from build123d import *

# Parameters (mm, degrees)
BOSS_EXTRUDE1_DEPTH     = 12.7
FILLET2_SIZE            = 41.275
FILLET2_SIZE_2          = 69.85
FILLET3_R               = 25.4
FILLET4_R               = 19.05
FILLET5_START           = -1
FILLET5_DEPTH           = 15
FILLET6_R               = 127
CUT_EXTRUDE1_REACH      = 634.314
SKETCH3_W               = 241.600142069
SKETCH3_H               = 584.2
F_8_CLEARANCE_HOLE1_D   = 4.9149
F_1_4_CLEARANCE_HOLE1_D = 7.14248


with BuildPart() as part:
    # Sketch1 → Boss-Extrude1 (new body)
    with BuildSketch(Plane.XY):
        Polygon((-228.088766336, 0), (228.088766336, 0), (228.088766336, -443.878997916), (241.600142069, -584.2), (237.284597128, -584.2), (202.688766336, -463.55), (79.375, -463.55), (79.375, -363.22), (-79.375, -363.22), (-79.375, -463.55), (-202.688766336, -463.55), (-237.284597128, -584.2), (-241.600142069, -584.2), (-228.088766336, -443.878997916), align=None)
    extrude(amount=BOSS_EXTRUDE1_DEPTH)

    # Fillet2
    # a fillet whose section is not a circle: 69.85, 41.275 mm, written as the material it adds along each edge
    with BuildSketch(Plane(origin=(-79.375, -363.22, 0), x_dir=(1, 0, 0), z_dir=(0, 0, 1))) as fillet2_piece_1:
        with BuildLine():
            Bezier((FILLET2_SIZE, 0), (0, 0), (0, -FILLET2_SIZE_2), weights=[1, 1.5, 1])
            Line((0, -FILLET2_SIZE_2), (0, 0))
            Line((0, 0), (FILLET2_SIZE, 0))
        make_face()
    extrude(amount=12.7)

    # Fillet3
    fillet3_edges = [part.edges().sort_by_distance(p)[0] for p in [
        (-79.375, -463.55, 6.35),
    ]]
    fillet(fillet3_edges, radius=FILLET3_R)

    # Fillet4
    fillet4_edges = [part.edges().sort_by_distance(p)[0] for p in [
        (-202.688766336, -463.55, 6.35),
    ]]
    fillet(fillet4_edges, radius=FILLET4_R)

    # Fillet5: read off the stored shape, not the designer's step
    # Fillet5 outline → Fillet5 (cut)
    with BuildSketch(Plane.XY.offset(FILLET5_START)):
        with BuildLine():
            Line((-237.284597128, -584.2), (-224.526592015, -539.707548693))
            add(Edge.make_bspline(
                [(-224.526592015, -539.707548693), (-237.177095318, -583.825096633), (-241.600142069, -584.2)],
                knots=[0, 0, 0, 1, 1, 1], degree=2, weights=[1, 2.333333333, 1]))
            Line((-241.600142069, -584.2), (-237.284597128, -584.2))
        make_face()
    extrude(amount=FILLET5_DEPTH, mode=Mode.SUBTRACT)

    # Fillet6
    # the kernel refuses this fillet: 127 mm, written as the material it adds along each edge
    with BuildSketch(Plane(origin=(-228.088766336, -443.878997916, 0), x_dir=(0, 1, 0), z_dir=(0, 0, 1))) as fillet6_piece_1:
        with BuildLine():
            CenterArc((FILLET6_R * 0.0480334444852, FILLET6_R), FILLET6_R, 264.5, 5.5)
            Line((-FILLET6_R * 0.047812308035, FILLET6_R * 0.00460380163282), (0, 0))
            Line((0, 0), (FILLET6_R * 0.0480334444852, 0))
        make_face()
    extrude(amount=12.7)

    # Sketch3 → Cut-Extrude1 (cut, up to next)
    with BuildSketch(Plane.XY.offset(12.7), mode=Mode.PRIVATE) as cut_extrude1_sk1:
        with Locations((120.800071035, -292.1)):
            Rectangle(SKETCH3_W, SKETCH3_H)
    cut_extrude1_tool1 = extrude(cut_extrude1_sk1.sketch, amount=-CUT_EXTRUDE1_REACH, mode=Mode.PRIVATE) & part.part
    add(cut_extrude1_tool1.solids().sort_by_distance((120.800071, -292.1, 12.7))[0], mode=Mode.SUBTRACT)

    # Mirror5: part across plane


with BuildPart() as part_1:
    add(part.part)
    add(part.part.mirror(Plane(origin=(0, 0, -0.35025), x_dir=(0, 0, 1), z_dir=(-1, 0, 0))))

    # #8 Clearance Hole1 (through all)
    with Locations(Plane(origin=(0, 0, 0), x_dir=(-1, 0, 0), z_dir=(0, 0, -1))):
        with Locations((12.077216058, -342.5825), (-12.077216058, -342.5825)):
            Hole(F_8_CLEARANCE_HOLE1_D / 2)

    # 1/4 Clearance Hole1 (through all)
    with Locations(Plane(origin=(0, 0, 0), x_dir=(-1, 0, 0), z_dir=(0, 0, -1))):
        with Locations((0, -352.7425), (0, -332.4225)):
            Hole(F_1_4_CLEARANCE_HOLE1_D / 2)


solid = part_1.part
Input: part model. Units: mm. Frame: model coordinates. A direction names the side the tool comes from. Coordinates: 2 decimals unless noted, no trailing zeros. Order: outer loops, then holes, each group sorted by start corner. A loop starts at its lowest first (then second) coordinate and runs counter-clockwise, first axis right, second up. Notation, with made-up numbers: M 30,56.25 L 43,56.25 A24 cw 43,85.25 Z; hole C 72,-39 d7. An arc over 180 degrees is marked long. Answer as CSV lines item,"result".
1. Access query for faces 4 (the cylindrical face through (199.66, -467.283, 6.439)), 5 (the flat face through (228.089, -222, 6)), 6 (the flat face through (3, -223, 0)). Directions: +Z, -Z, +X, -X, +Y, -Y. A direction counts if a zero-diameter tool reaches every point of the face in a straight line with its end or side. Return the directions, or none.
Reported:
face 4,"+Z, -Z, -Y"
face 5,"+Z, -Z, +X, +Y"
face 6,"-Z, +X, -X, +Y, -Y"
2. Section A-A (y = -457). Return the cut outline in (x, z).
Reported:
outline,"M -229.35,0 L -87.75,0 L -87.75,12.7 L -229.35,12.7 Z; M 87.75,0 L 229.35,0 L 229.35,12.7 L 87.75,12.7 Z"
3. Section D-D (z = 7.5). State how many separate pieces and enclosed holes the cut face has, then the cut area to 3 significant figures.
Reported:
separate pieces,"1"
enclosed holes,"4"
area,"200,000 mm2"
4. Material intervals for line 1 (X direction, y = -93, z = 10.75); line 2 (Y direction, x = -116, z = 12); line 3 (X direction, y = -420, z = 3.75), sorted ascending. Write a range as from..to.
Reported:
line 1,"-228.09..228.09"
line 2,"-463.55..0"
line 3,"-228.09..-79.19, 79.19..228.09"
5. First-contact query: P1, Ø3, axis at x = -109.5, z = 2.5, coming from the +Y side; P2, Ø4, axis at y = -82, z = 4.5, coming from the -X side; P3, Ø3, axis at x = 151, z = 7, coming from the -Y side; P4, Ø4, axis at y = -174.5, z = 3.5, coming from the +X side. Flat tips, straight axial feed; report the tip coordinate or a pass-through.
Reported:
P1,"y = 0"
P2,"x = -228.09"
P3,"y = -463.55"
P4,"x = 228.09"
6. Section B-B (y = -193.5). Return the cut outline in (x, z), then the cut area to 3 significant figures.
Reported:
outline,"M -228.09,0 L 228.09,0 L 228.09,12.7 L -228.09,12.7 Z"
area,"5,790 mm2"
7. Pull-direction query (X, two-part tool) for faces 1 (the cylindrical face through (228.24, -443.96, 6.26)), 2 (the flat face through (-228.089, -222, 6)), 3 (the cylindrical face through (-86.618, -455.912, 6.439)); classes: released by +X, released by -X, zero draft, split by the parting line, or undercut.
Reported:
face 1,"released by +X"
face 2,"released by -X"
face 3,"undercut"
8. Section C-C (x = -145). Return the cut outline in (y, z), then the cut area to 3 significant figures.
Reported:
outline,"M -463.55,0 L 0,0 L 0,12.7 L -463.55,12.7 Z"
area,"5,890 mm2"
